Design review of the part built by this model. Coordinates are the model's own, in mm. A direction names the side the tool comes from. Give positions to 0.01 mm unless a question says otherwise; leave off trailing zeros. Loops run counter-clockwise (first coordinate to the right, second up) from the corner with the lowest first, then second, coordinate; pieces in that order, holes last. Notation, with made-up numbers: (-10.75, 69.25) -> (1.25, 69.25) arc R22 ccw to (1.25, 92.25) -> close; hole circle Ø1 at (65, 59). An arc over 180 degrees is marked (long way). Use a Markdown table: item, result. Add a question column.
1. Add section A-A (x = 78.75). State the section outline as (y, z) points, and give its area (3 significant figures).
2. To check wall thickness, follow line 1 (Z direction, x = 74.5, y = -38.5); line 2 (X direction, y = 2, z = -61); line 3 (Z direction, x = 83.75, y = 5). State the ranges of each line that lie inside material, in increasing order.
3. Draft analysis for pull direction Z (two halves, no side actions). For faces 5 (the flat face through (77, 37.75, -57)), 6 (the flat face through (84.537, -0.14, -26.431)), 7 (the flat face through (72, -40, -52)), state which applies: pulls with the +Z half, pulls with the -Z half, needs draft (parallel to the pull), parting line crosses it, or undercut.
4. For pin 1 Ø3.5 at (x, z) = (76.5, -58) entering from +Y; pin 2 Ø8 at (x, z) = (80.5, -52.5) entering from +Y; pin 3 Ø12 at (x, z) = (79, -54) entering from +Y; pin 4 Ø4.5 at (x, z) = (77, -41.5) entering from -Y, all flat-tipped, find the tip position at first contact; note any pin that passes through.
5. For faces 1 (the flat face through (73.174, -36.736, -56.807)), 2 (the flat face through (72, -40, -61.75)), 3 (the flat face through (83.3, -24.9, -26)), 4 (the flat face through (67.82, 41.844, -56.807)), list the 3-axis set-ups (+Z, -Z, +X, -X, +Y, -Y) from which the entire face can be reached by the end or side of a thin tool; tool diameter is ignored.
6. Add section C-C (z = -49.5). State the section outline as (x, y) points, and give its area (3 significant figures).
```python
from build123d import *

# Parameters (mm, degrees)
EXTRUDE136083_DEPTH                     = 20
EXTRUDE136083_ONTO_SKETCH302_ROLL_ANGLE = 90
EXTRUDE136073_DEPTH                     = 9.75
BOX023_W                                = 25
BOX023_H                                = 80
BOX023_DEPTH                            = 51
EXTRUDE136056_DEPTH                     = 40
EXTRUDE136055_DEPTH                     = 42
FILLET007_R                             = 2


with BuildPart() as extrude136083:
    # Sketch302 as drawn → Extrude136083 (new)
    with BuildSketch(Plane.XY):
        Polygon((2, -3.464102), (0, 0), (1.03923, 0.6), (2, 0.6), align=None)
    extrude(amount=-EXTRUDE136083_DEPTH)


with BuildPart() as extrude136083_1:
    # Extrude136083 onto Sketch302 roll: moved
    add(extrude136083.part.rotate(Axis((0, 0, 0), (1, 0, 0)), EXTRUDE136083_ONTO_SKETCH302_ROLL_ANGLE))


with BuildPart() as extrude136083_2:
    # Extrude136083 onto Sketch302 placement: moved
    add(extrude136083_1.part.moved(Location((0, -10, 0))))


with BuildPart() as extrude136083_3:
    # Extrude136083 placement: moved
    add(extrude136083_2.part.moved(Location((84, 0, 0))))


with BuildPart() as fusion034004041072:
    # Sketch294 → Extrude136073 (new body)
    with BuildSketch(Plane.XY):
        Polygon((-1, 35.75), (0, 35.75), (0.352654, 37.75), (8.25, 37.75), (8.25, 40), (2.25, 40), (-2.699747, 44.949747), (-6.285534, 44.949747), (-6.285534, 42.949747), (-4.042893, 40.707107), (-4.75, 40), (-4.75, 38.375778), align=None)
        Polygon((-1, -35.75), (0, -35.75), (0.352654, -37.75), (8.25, -37.75), (8.25, -40), (2.25, -40), (-2.699747, -44.949747), (-6.285534, -44.949747), (-6.285534, -42.949747), (-4.042893, -40.707107), (-4.75, -40), (-4.75, -38.375778), align=None)
    extrude(amount=-EXTRUDE136073_DEPTH)


with BuildPart() as fusion034004041072_1:
    # Extrude136073 placement: moved
    add(fusion034004041072.part.moved(Location((73, 0, -26.5))))

    # Fusion034004041072: union Extrude136083
    add(extrude136083_3.part)


with BuildPart() as cube020:
    # Box023 → Box023 (new body)
    with BuildSketch(Plane(origin=(80.25, -40, -51.5), x_dir=(1, 0, 0), z_dir=(0, 0, 1))):
        with Locations((12.5, 40)):
            Rectangle(BOX023_W, BOX023_H)
    extrude(amount=BOX023_DEPTH)


with BuildPart() as extrude136056:
    # Sketch277 → Extrude136056 (new body)
    with BuildSketch(Plane.XY):
        with BuildLine():
            ThreePointArc((81.0383, -34.5), (85.059706, 0), (81.0383, 34.5))
            Line((66.5383, 34.5), (81.0383, 34.5))
            Line((63.0383, 38), (66.5383, 34.5))
            Line((40.0383, 38), (63.0383, 38))
            Line((27.5383, 25.5), (40.0383, 38))
            Line((12.636376, 25.5), (27.5383, 25.5))
            Line((10.0383, 30), (12.636376, 25.5))
            Line((10.0383, 30), (-52.9617, 30))
            Line((-62.9617, 26), (-52.9617, 30))
            Line((-82.9617, 25), (-62.9617, 26))
            ThreePointArc((-82.9617, 25), (-85.059706, 0), (-82.9617, -25))
            Line((-82.9617, -25), (-62.9617, -26))
            Line((-62.9617, -26), (-52.9617, -30))
            Line((10.0383, -30), (-52.9617, -30))
            Line((10.0383, -30), (12.636376, -25.5))
            Line((12.636376, -25.5), (27.5383, -25.5))
            Line((27.5383, -25.5), (40.0383, -38))
            Line((40.0383, -38), (63.0383, -38))
            Line((63.0383, -38), (66.5383, -34.5))
            Line((66.5383, -34.5), (81.0383, -34.5))
        make_face()
    extrude(amount=-EXTRUDE136056_DEPTH)


with BuildPart() as batterycoverfillet007:
    # Sketch276 → Extrude136055 (new body)
    with BuildSketch(Plane.XY):
        with BuildLine():
            ThreePointArc((-84.489299, 32), (-87.942378, 0), (-84.489299, -32))
            Line((-84.489299, -32), (29.510701, -32))
            Line((29.510701, -32), (37.510701, -40))
            Line((37.510701, -40), (82.510701, -40))
            ThreePointArc((82.510701, -40), (87.942378, 0), (82.510701, 40))
            Line((37.510701, 40), (82.510701, 40))
            Line((29.510701, 32), (37.510701, 40))
            Line((-84.489299, 32), (29.510701, 32))
        make_face()
    extrude(amount=-EXTRUDE136055_DEPTH)

    # Cut009010006006006005016: cut Extrude136056
    add(extrude136056.part, mode=Mode.SUBTRACT)

    # Common001: intersect Cube020
    add(cube020.part, mode=Mode.INTERSECT)

    # Fusion034004041073: union Fusion034004041072
    add(fusion034004041072_1.part)

    # Fillet007
    fillet007_edges = [batterycoverfillet007.edges().sort_by_distance(p)[0] for p in [
        (81.380351, 40, -42),
        (87.942378, 0, -42),
        (81.380351, -40, -42),
        (82.510701, 40, -21.25),
        (87.942378, 0, -0.5),
        (82.510701, -40, -21.25),
    ]]
    fillet(fillet007_edges, radius=FILLET007_R)


with BuildPart() as batterycoverfillet007_1:
    # Fillet007 placement: moved
    add(batterycoverfillet007.part.moved(Location((0, 0, -25.5))))


solid = batterycoverfillet007_1.part
```
Taken from the geometry:
| question | item | result |
|---|---|---|
| 1 | outline | (-40, -61.75) -> (-37.75, -61.75) -> (-37.75, -52) -> (-40, -52) -> close; (37.75, -61.75) -> (40, -61.75) -> (40, -52) -> (37.75, -52) -> close |
| 1 | area | 43.9 mm^2 |
| 2 | line 1 | z = -61.75 to -52 |
| 2 | line 2 | x = 85.05 to 87.93 |
| 2 | line 3 | z = -67.5 to -65.5 |
| 3 | face 5 | needs draft |
| 3 | face 6 | undercut |
| 3 | face 7 | pulls with the +Z half |
| 4 | pin 1 | stops at y = 40.5 |
| 4 | pin 2 | stops at y = 40 |
| 4 | pin 3 | stops at y = 42.25 |
| 4 | pin 4 | passes through |
| 5 | face 1 | +Z, -Z |
| 5 | face 2 | -Z, -X, +Y, -Y |
| 5 | face 3 | +Z, +X, -X, -Y |
| 5 | face 4 | +Z, -Z, -X |
| 6 | outline | (80.25, -40) -> (80.98, -40) arc R2 ccw to (82.91, -38.51) arc R150 ccw to (82.91, 38.51) arc R2 ccw to (80.98, 40) -> (80.25, 40) -> (80.25, 34.5) -> (81.04, 34.5) arc R150 cw to (81.04, -34.5) -> (80.25, -34.5) -> close |
| 6 | area | 231 mm^2 |
